Could you check a few things on this drawing? It's one solid part, dimensions in mm from its lowest x, y, z. A direction names the side the tool comes from. Round coordinates to 2 decimals unless told otherwise and drop trailing zeros. Write each loop counter-clockwise with the first axis right and the second up, starting at its lowest first coordinate (ties: lowest second). Pieces come first, ordered by that corner, then holes. Notation, with made-up numbers: M 79,-26.5 L 85,-26.5 A15 cw 85,-15.5 Z; hole C 25,23 d11. An arc over 180 degrees is marked long. One line per question, with ' | ' between items. Start each with the question number.
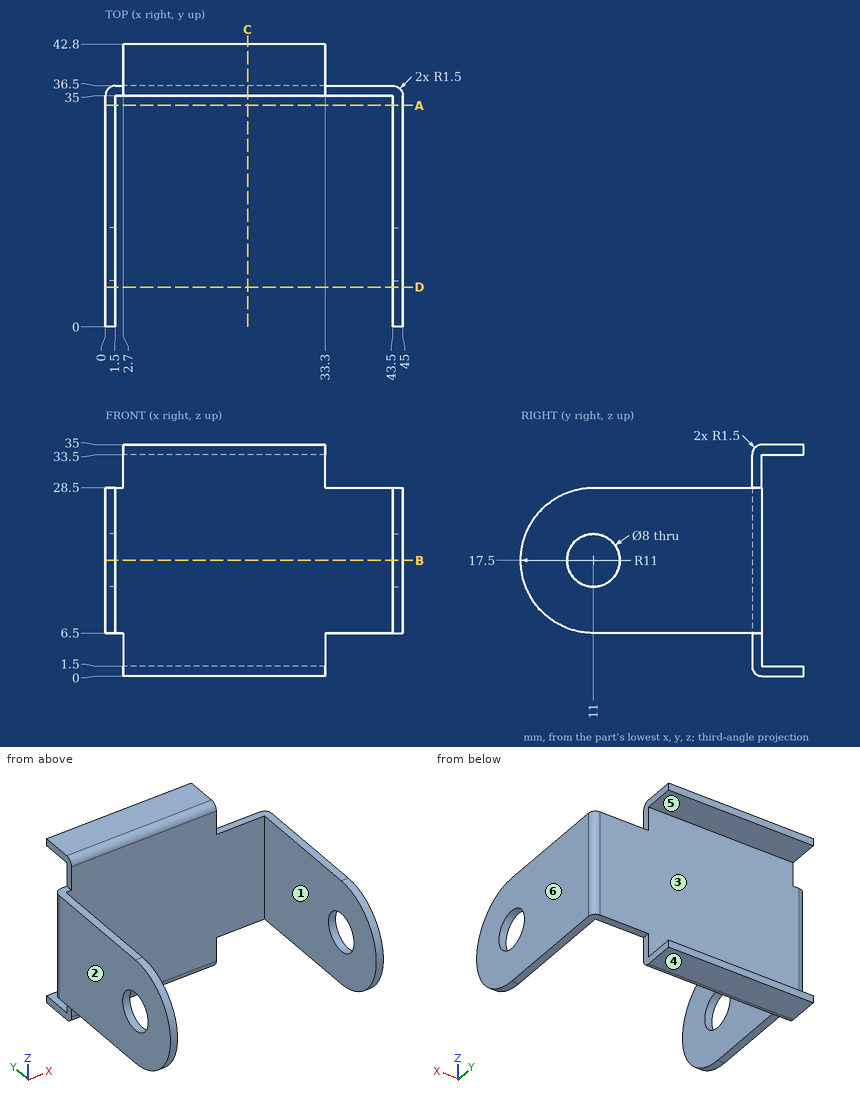
1. Suppose I cut it at C-C (x = 21.5). Write out the boundary of the cut face in (y, z), and give its area (3 significant figures).
2. I need wall thicknesses on line 1 along X through (y, z) = (27.5, 20); line 2 along Z through (x, y) = (22, 40.5); line 3 along Y through (x, z) = (0.7, 17.5). Which ranges of each line are inside material? Lowest first, please. Write a range as from..to.
3. Suppose I cut it at B-B (z = 17.5). Write out the boundary of the cut face in (x, y), and give its area (3 significant figures).
4. Suppose I cut it at A-A (y = 33.5). Write out the boundary of the cut face in (x, z), and give its area (3 significant figures).
5. If we mould it in two halves opening along Z, with no side actions, what happens to the marked faces 3, 4, 5 and 6? For each: released by +Z, released by -Z, zero draft, split by the parting line, or undercut.
6. I'm going to push flat-ended pins straight in: P1, Ø5, axis at y = 11, z = 17.5, coming from the -X side; P2, Ø7, axis at y = 37.5, z = 4.5, coming from the +X side; P3, Ø3, axis at x = 22, z = 3.5, coming from the -Y side; P4, Ø2, axis at x = 1.5, y = 20.5, coming from the +Z side. Where does each tip first touch, or does it pass through?
7. Which directions (+Z, -Z, +X, -X, +Y, -Y) give clear straight access to the entire face, cutting with the end or side of a thin tool? Please do the marked faces 1 and 2.
8. Suppose I cut it at D-D (y = 6). Write out the boundary of the cut face in (x, z).
Computed:
1) outline: M 35,1.5 A1.5 ccw 36.5,0 L 42.8,0 L 42.8,1.5 L 36.5,1.5 L 36.5,33.5 L 42.8,33.5 L 42.8,35 L 36.5,35 A1.5 ccw 35,33.5 Z | area: 70.4 mm²
2) line 1: x = 0..1.5, 43.5..45 | line 2: z = 0..1.5, 33.5..35 | line 3: y = 0..7, 15..36.27
3) outline: M 0,0 L 1.5,0 L 1.5,7 L 0,7 Z; M 0,15 L 1.5,15 L 1.5,35 L 43.5,35 L 43.5,15 L 45,15 L 45,35 A1.5 ccw 43.5,36.5 L 1.5,36.5 A1.5 ccw 0,35 Z; M 43.5,0 L 45,0 L 45,7 L 43.5,7 Z | area: 148 mm²
4) outline: M 0,6.5 L 1.5,6.5 L 1.5,28.5 L 0,28.5 Z; M 43.5,6.5 L 45,6.5 L 45,28.5 L 43.5,28.5 Z | area: 66.0 mm²
5) face 3: undercut | face 4: released by -Z | face 5: undercut | face 6: zero draft
6) P1: passes through | P2: stops at x = 45 | P3: stops at y = 35 | P4: stops at z = 28.5
7) face 1: +Z, -Z, -Y | face 2: +Z, -Z, -X, +Y, -Y
8) outline: M 0,7.7 L 1.5,7.7 L 1.5,27.3 L 0,27.3 Z; M 43.5,7.7 L 45,7.7 L 45,27.3 L 43.5,27.3 Z
